from build123d import *

# Parameters (mm, degrees)
F0_W      = 90
F0_H      = 50
F1_DEPTH  = 2
F3_R      = 5.08
F4_R      = 5.08
F5_R      = 5.08
F6_R      = 5.08
F8_W      = 10
F8_H      = 4
F9_DEPTH  = 25.4
F10_R     = 1.5
F11_DEPTH = 25.4
F12_R     = 3
F13_DEPTH = 25.4


with BuildPart() as f1:
    # F0 (on Top) → F1 (new body)
    with BuildSketch(Plane.XY):
        with Locations((45, 25)):
            Rectangle(F0_W, F0_H)
    extrude(amount=F1_DEPTH)

    # F3
    f3_edges = [f1.edges().sort_by_distance(p)[0] for p in [
        (90, 0, 1),
    ]]
    fillet(f3_edges, radius=F3_R)

    # F4
    f4_edges = [f1.edges().sort_by_distance(p)[0] for p in [
        (90, 50, 1),
    ]]
    fillet(f4_edges, radius=F4_R)

    # F5
    f5_edges = [f1.edges().sort_by_distance(p)[0] for p in [
        (0, 50, 1),
    ]]
    fillet(f5_edges, radius=F5_R)

    # F6
    f6_edges = [f1.edges().sort_by_distance(p)[0] for p in [
        (0, 0, 1),
    ]]
    fillet(f6_edges, radius=F6_R)

    # F8 (on offset) → F9 (cut)
    with BuildSketch(Plane.XY.offset(2)):
        with BuildLine():
            Line((35, 22.5), (35, 27.5))
            Line((35, 27.5), (35.8850657517, 27.5))
            add(Edge.make_bspline(
                [(35.8850657517, 27.5), (29.9931568267, 28.0368228686), (29.9931568267, 25)],
                knots=[4.5346839474, 4.5346839474, 4.5346839474, 6.2831853072, 6.2831853072, 6.2831853072], degree=2, weights=[1, 0.6415718139, 1]))
            add(Edge.make_bspline(
                [(29.9931568267, 25), (29.9931568267, 21.9631771314), (35.8850657517, 22.5)],
                knots=[0, 0, 0, 1.7485013598, 1.7485013598, 1.7485013598], degree=2, weights=[1, 0.6415718139, 1]))
            Line((35.8850657517, 22.5), (35, 22.5))
        make_face()
        with BuildLine():
            Line((35.8850657517, 27.5), (35, 27.5))
            Line((35, 27.5), (35, 22.5))
            Line((35, 22.5), (35.8850657517, 22.5))
            add(Edge.make_bspline(
                [(35.8850657517, 22.5), (40.0068431733, 22.8755428686), (40.0068431733, 25), (40.0068431733, 27.1244571314), (35.8850657517, 27.5)],
                knots=[1.7485013598, 1.7485013598, 1.7485013598, 3.1415926536, 3.1415926536, 4.5346839474, 4.5346839474, 4.5346839474], degree=2, weights=[1, 0.767062975, 1, 0.767062975, 1]))
        make_face()
        with BuildLine():
            Line((50, 27.5), (35.8850657517, 27.5))
            add(Edge.make_bspline(
                [(35.8850657517, 22.5), (40.0068431733, 22.8755428686), (40.0068431733, 25), (40.0068431733, 27.1244571314), (35.8850657517, 27.5)],
                knots=[1.7485013598, 1.7485013598, 1.7485013598, 3.1415926536, 3.1415926536, 4.5346839474, 4.5346839474, 4.5346839474], degree=2, weights=[1, 0.767062975, 1, 0.767062975, 1]))
            Line((35.8850657517, 22.5), (50, 22.5))
            Line((50, 22.5), (50, 27.5))
        make_face()
        with Locations((45, 30.5)):
            Rectangle(F8_W, F8_H)
        Polygon((40, 28.5), (40, 32.5), (35, 28.5), align=None)
        Polygon((35, 21.5), (40, 17.5), (40, 21.5), align=None)
        with Locations((45, 19.5)):
            Rectangle(F8_W, F8_H)
        with BuildLine():
            Line((58.6482731998, 30.5), (53, 32.5))
            ThreePointArc((53, 32.5), (51.4781820371, 30.5), (53, 28.5))
            Line((53, 28.5), (58.6482731998, 30.5))
        make_face()
        with BuildLine():
            ThreePointArc((53, 21.5), (51.4781820371, 19.5), (53, 17.5))
            Line((53, 17.5), (58.6482731998, 19.5))
            Line((58.6482731998, 19.5), (53, 21.5))
        make_face()
    extrude(amount=-F9_DEPTH, mode=Mode.SUBTRACT)

    # F10 (on offset) → F11 (cut)
    with BuildSketch(Plane.XY.offset(2)):
        with Locations((23.6474, 3)):
            Circle(F10_R)
        with Locations((66.3526, 3)):
            Circle(F10_R)
        with Locations((23.6474, 47)):
            Circle(F10_R)
        with Locations((66.3526, 47)):
            Circle(F10_R)
    extrude(amount=-F11_DEPTH, mode=Mode.SUBTRACT)

    # F12 (on offset) → F13 (cut)
    with BuildSketch(Plane.XY.offset(2)):
        with Locations((15.6768597662, 33.8291116059)):
            Circle(F12_R)
    extrude(amount=-F13_DEPTH, mode=Mode.SUBTRACT)


solid = f1.part
Design review of the part built by this model. Coordinates are the model's own, in mm. A direction names the side the tool comes from. Coordinates: 2 decimals unless noted, no trailing zeros. Loops run counter-clockwise (first coordinate to the right, second up) from the corner with the lowest first, then second, coordinate; pieces in that order, holes last. Notation, with made-up numbers: M 27.25,-6 L 66.25,-6 A21 ccw 66.25,18 Z; hole C 33.25,27.25 d7. An arc over 180 degrees is marked long. Use one line per item in the form item = value.
(1) For line 1 along Y through (x, z) = (48, 1.7); line 2 along X through (y, z) = (47.5, 1.75); line 3 along Y through (x, z) = (37.5, 0.75), list the stretches that pass through material, from the lowest coordinate up. Write a range as from..to.
Return value:
line_1 = 0..17.5, 21.5..22.5, 27.5..28.5, 32.5..50
line_2 = 0.7..22.23, 25.06..64.94, 67.77..89.3
line_3 = 0..19.5, 21.5..22.5, 27.5..28.5, 30.5..50
(2) For faces 1 (the face through (45, 17.5, 1)), 2 (the face through (90, 25, 1)), list the 3-axis set-ups (+Z, -Z, +X, -X, +Y, -Y) from which the entire face can be reached by the end or side of a thin tool; tool diameter is ignored.
Return value:
face_1 = +Z, -Z
face_2 = +Z, -Z, +X, +Y, -Y
(3) Consider section A-A (x = 47). Write out the cut boundary in (y, z).
Return value:
outline = M 0,0 L 17.5,0 L 17.5,2 L 0,2 Z; M 21.5,0 L 22.5,0 L 22.5,2 L 21.5,2 Z; M 27.5,0 L 28.5,0 L 28.5,2 L 27.5,2 Z; M 32.5,0 L 50,0 L 50,2 L 32.5,2 Z
(4) Consider section D-D (z = 1.6). Give the number of separate pieces and of enclosed holes in the cut face, and give its area (3 significant figures).
Return value:
separate_pieces = 1
enclosed_holes = 10
area = 4,190 mm2
(5) Draft analysis for pull direction Y (two halves, no side actions). For faces 3 (the face through (50, 19, 1)), 4 (the face through (54, 25, 0)), 5 (the face through (44, 50, 1)), state which applies: pulls with the +Y half, pulls with the -Y half, needs draft (parallel to the pull), parting line crosses it, or undercut.
Return value:
face_3 = undercut
face_4 = needs draft
face_5 = pulls with the +Y half
(6) Consider section B-B (y = 47). Write out the cut boundary in (x, z), and give its area (3 significant figures).
Return value:
outline = M 0.45,0 L 22.15,0 L 22.15,2 L 0.45,2 Z; M 25.15,0 L 64.85,0 L 64.85,2 L 25.15,2 Z; M 67.85,0 L 89.55,0 L 89.55,2 L 67.85,2 Z
area = 166 mm2
(7) Consider section C-C (y = 35). Write out the cut boundary in (x, z).
Return value:
outline = M 0,0 L 12.91,0 L 12.91,2 L 0,2 Z; M 18.44,0 L 90,0 L 90,2 L 18.44,2 Z
